Could you check a few things on this model? Use its own coordinates, in mm. A direction names the side the tool comes from. Round coordinates to 2 decimals unless told otherwise and drop trailing zeros. Write each loop counter-clockwise with the first axis right and the second up, starting at its lowest first coordinate (ties: lowest second). Pieces come first, ordered by that corner, then holes. Notation, with made-up numbers: (54, -27) -> (61, -27) arc R20 cw to (61, -15) -> close; hole circle Ø11 at (13.5, 30). An arc over 180 degrees is marked (long way). Answer in a Markdown table with one row per item. Add a question column.
```python
from build123d import *

# Parameters (mm, degrees)
F0_W      = 127
F0_H      = 127
F1_DEPTH  = 25.4
F2_R      = 3.81
F3_DEPTH  = 7.62
F4_R      = 5.08
F5_R      = 5.08
F6_R      = 5.08
F7_R      = 5.08
F8_R      = 5.08
F9_R      = 3.81
F10_DEPTH = 12.7
F11_R     = 3.81
F12_DEPTH = 12.7


with BuildPart() as f1:
    # F0 (on Top) → F1 (new body)
    with BuildSketch(Plane.XY):
        with Locations((-4.09049, 24.324038)):
            Rectangle(F0_W, F0_H)
    extrude(amount=F1_DEPTH)

    # F2 (on face) → F3 (join)
    with BuildSketch(Plane.XY.offset(25.4)):
        with Locations((-55.712551, 73.958889)):
            Circle(F2_R)
    extrude(amount=F3_DEPTH)

    # F4
    f4_edges = [f1.edges().sort_by_distance(p)[0] for p in [
        (59.40951, 24.324038, 25.4),
    ]]
    fillet(f4_edges, radius=F4_R)

    # F5
    f5_edges = [f1.edges().sort_by_distance(p)[0] for p in [
        (-6.63049, -39.175962, 25.4),
    ]]
    fillet(f5_edges, radius=F5_R)

    # F6
    f6_edges = [f1.edges().sort_by_distance(p)[0] for p in [
        (-67.59049, 26.864038, 25.4),
    ]]
    fillet(f6_edges, radius=F6_R)

    # F7
    f7_edges = [f1.edges().sort_by_distance(p)[0] for p in [
        (-4.09049, 87.824038, 25.4),
    ]]
    fillet(f7_edges, radius=F7_R)

    # F8
    f8_edges = [f1.edges().sort_by_distance(p)[0] for p in [
        (59.40951, 24.324038, 0),
    ]]
    fillet(f8_edges, radius=F8_R)

    # F9 (on face) → F10 (join)
    with BuildSketch(Plane.XZ.offset(39.175962)):
        with Locations((32.560311, 13.580429)):
            Circle(F9_R)
    extrude(amount=F10_DEPTH)

    # F11 (on face) → F12 (join)
    with BuildSketch(Plane(origin=(0, 87.824038, 0), x_dir=(-1, 0, 0), z_dir=(0, 1, 0))):
        with Locations((-40.414046, 11.944233)):
            Circle(F11_R)
    extrude(amount=F12_DEPTH)


solid = f1.part
```
(1) Suppose I cut it at A-A, the plane y = -32. Please give me the cut outline in (x, z), then the cut area to 3 significant figures.
(2) On a 3-axis mill with a long thin cutter (end or side, diameter ignored), from which of +Z, -Z, +X, -X, +Y, -Y can I reach the whole of each face in a straight line? I mean faces 1 (the face through (-66.06, 86.38, 12.81)), 2 (the face through (-52.193, 72.5, 29.157)), 3 (the face through (44.22, 94.09, 12.11)). Say none if no direction works.
(3) For P1, Ø12, axis at x = 20, z = 14.5, coming from the -Y side; P2, Ø12, axis at x = -52.5, y = -24, coming from the +Z side; P3, Ø4, axis at x = -7.5, z = 27, coming from the -Y side, each with a flat end and sliding along its axis, tell me the tip position at first contact or that it passes through.
(4) Suppose I cut it at D-D, the plane z = 30. Please give me the cut outline in (x, y), then the cut area to 3 significant figures.
(5) Suppose I cut it at C-C, the plane x = 34. Please give me the cut outline in (y, z).
(6) Suppose I cut it at B-B, the plane x = 48. Please give me the cut outline in (y, z).
(7) I need wall thicknesses on L1, parallel to Y at x = -29.5, z = 8; L2, parallel to Z at x = -34.5, y = 50; L3, parallel to X at y = -22.5, z = 20.5. Which ranges of each line are inside material? Lowest first, please.
Response:
| question | item | result |
|---|---|---|
| 1 | outline | (-67.59, 5.08) arc R5.08 ccw to (-62.51, 0) -> (54.33, 0) arc R5.08 ccw to (59.41, 5.08) -> (59.41, 20.32) arc R5.08 ccw to (54.33, 25.4) -> (-62.51, 25.4) arc R5.08 ccw to (-67.59, 20.32) -> close |
| 1 | area | 3,200 mm² |
| 2 | face 1 | +Z, -Z, -X, +Y |
| 2 | face 2 | +Z |
| 2 | face 3 | +Y |
| 3 | P1 | y = -39.18 |
| 3 | P2 | z = 25.4 |
| 3 | P3 | y = -36.07 |
| 4 | outline | circle Ø7.62 at (-55.71, 73.96) |
| 4 | area | 45.6 mm² |
| 5 | outline | (-51.88, 10.05) -> (-39.18, 10.05) -> (-39.18, 5.08) arc R5.08 ccw to (-34.1, 0) -> (82.74, 0) arc R5.08 ccw to (87.82, 5.08) -> (87.82, 20.32) arc R5.08 ccw to (82.74, 25.4) -> (-34.1, 25.4) arc R5.08 ccw to (-39.18, 20.32) -> (-39.18, 17.11) -> (-51.88, 17.11) -> close |
| 6 | outline | (-39.18, 5.08) arc R5.08 ccw to (-34.1, 0) -> (82.74, 0) arc R5.08 ccw to (87.82, 5.08) -> (87.82, 20.32) arc R5.08 ccw to (82.74, 25.4) -> (-34.1, 25.4) arc R5.08 ccw to (-39.18, 20.32) -> close |
| 7 | L1 | -39.18 to 87.82 |
| 7 | L2 | 0 to 25.4 |
| 7 | L3 | -67.59 to 59.41 |
